Input: part model. Units: mm. Frame: model coordinates. Round coordinates to 2 decimals unless told otherwise and drop trailing zeros. Write each loop counter-clockwise with the first axis right and the second up, starting at its lowest first coordinate (ties: lowest second). Pieces come first, ordered by that corner, then holes. Notation, with made-up numbers: (26, 82.5) - (58, 82.5) arc R13 cw to (58, 96.5) - close; hole circle Ø8 at (13.25, 48). An arc over 180 degrees is marked (long way). One line per item, written item: value. Start each with the question number.
```python
from build123d import *

# Parameters (mm, degrees)
F1_DEPTH = 20
F2_R     = 1.5
F3_DEPTH = 25
F4_R     = 2.5
F5_DEPTH = 25
F6_DEPTH = 5


with BuildPart() as f1:
    # F0 (on Top) → F1 (new body)
    with BuildSketch(Plane.XY):
        Polygon((75, -10), (75, 0), (75, 10), (-75, 10), (-75, -10), align=None)
    extrude(amount=F1_DEPTH)

    # F2 (on face) → F3 (cut)
    with BuildSketch(Plane.XY.offset(20)):
        with Locations((-40, 0)):
            Circle(F2_R)
        with Locations((40, 0)):
            Circle(F2_R)
    extrude(amount=-F3_DEPTH, mode=Mode.SUBTRACT)

    # F4 (on face) → F5 (cut)
    with BuildSketch(Plane.XZ.offset(10)):
        with Locations((0, 10)):
            Circle(F4_R)
    extrude(amount=-F5_DEPTH, mode=Mode.SUBTRACT)

    # F6 (cut): a face of the model
    f6_faces = [f1.faces().sort_by_distance(p)[0] for p in [
        (-73.486725405, -10, 10),
    ]]
    extrude(f6_faces, amount=-F6_DEPTH, mode=Mode.SUBTRACT)


solid = f1.part
```
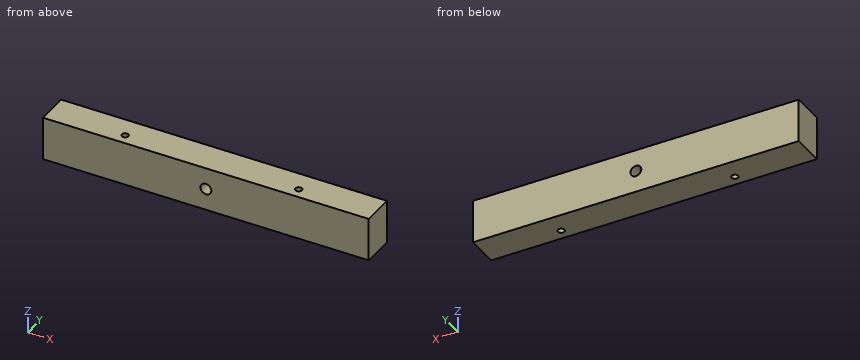
Q1. Material intervals for probe 1 along Z at (x, y) = (0, 5.75); probe 2 along Y at (x, z) = (-40, 13.5); probe 3 along X at (y, z) = (-0.5, 14), sorted ascending. Write a range as from..to.
Q2. Cut plane A-A, the plane x = 0. Output: boundary loops of the cut face in (y, z).
Q3. Contact query for a flat-ended pin moving along its axis: pin 1 Ø1.8 at (x, y) = (-40, 0) entering from -Z. Output: stop coordinate, or through.
A:
1. probe 1: z = 0..7.5, 12.5..20
1. probe 2: y = -5..-1.5, 1.5..10
1. probe 3: x = -75..-41.41, -38.59..38.59, 41.41..75
2. outline: (-5, 0) - (10, 0) - (10, 7.5) - (-5, 7.5) - close; (-5, 12.5) - (10, 12.5) - (10, 20) - (-5, 20) - close
3. pin 1: passes through
